from build123d import *

# Parameters (mm, degrees)
F0_W     = 75
F0_H     = 250
F1_DEPTH = 4
F2_W     = 40
F2_H     = 40
F3_DEPTH = 500
F4_W     = 30
F4_H     = 32
F5_DEPTH = 499
F6_R     = 5
F7_R     = 3
F9_DEPTH = 4


with BuildPart() as f1:
    # F0 (on Top) → F1 (new body)
    with BuildSketch(Plane.XY):
        with Locations((37.5, 125)):
            Rectangle(F0_W, F0_H)
    extrude(amount=F1_DEPTH)

    # F2 (on face) → F3 (join)
    with BuildSketch(Plane.XY.offset(4)):
        with Locations((37.5, 187.5)):
            Rectangle(F2_W, F2_H)
    extrude(amount=F3_DEPTH)

    # F4 (on face) → F5 (cut)
    with BuildSketch(Plane.XY.offset(504)):
        with Locations((37.5, 187.5)):
            Rectangle(F4_W, F4_H)
    extrude(amount=-F5_DEPTH, mode=Mode.SUBTRACT)

    # F6
    f6_edges = [f1.edges().sort_by_distance(p)[0] for p in [
        (57.5, 167.5, 254),
        (57.5, 207.5, 254),
        (17.5, 207.5, 254),
        (17.5, 167.5, 254),
    ]]
    fillet(f6_edges, radius=F6_R)

    # F7
    f7_edges = [f1.edges().sort_by_distance(p)[0] for p in [
        (0, 250, 2),
        (0, 0, 2),
        (75, 0, 2),
        (75, 250, 2),
    ]]
    fillet(f7_edges, radius=F7_R)

    # F8 (on face) → F9 (join)
    with BuildSketch(Plane.YZ.offset(57.5)):
        Polygon((172.5, 369.087671), (14.281406, 4), (44.281406, 4), (202.5, 369.087671), align=None)
    extrude(amount=F9_DEPTH)


solid = f1.part
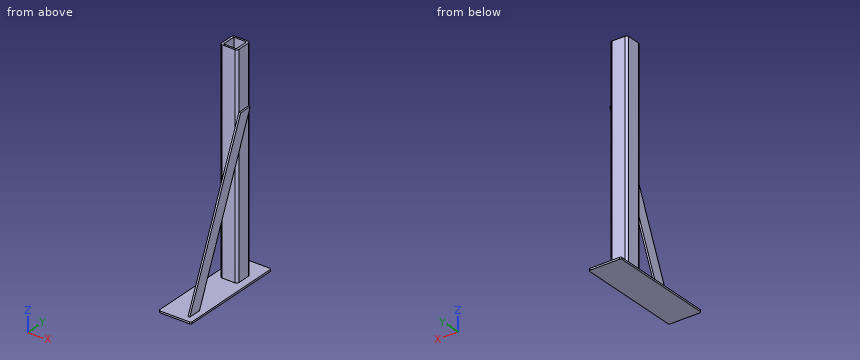
Could you check a few things on this model? Use its own coordinates, in mm. Round coordinates to 2 decimals unless told otherwise and drop trailing zeros. Loops run counter-clockwise (first coordinate to the right, second up) from the corner with the lowest first, then second, coordinate; pieces in that order, holes last. Notation, with made-up numbers: (22, 74) -> (65, 74) arc R31 ccw to (65, 110) -> close; hole circle Ø7 at (33, -31). An arc over 180 degrees is marked (long way). Use CSV: the item, a comma, the result in double quotes.
(1) If I drill on probe 1 along Y at (x, z) = (34, 323.5); probe 2 along Z at (x, y) = (51.5, 152.5); probe 3 along X at (y, z) = (58, 85), over which ranges is the centre line in solid material (lowest first)? Write a range as [from, to].
Return value:
probe 1,"y = [167.5, 171.5], [203.5, 207.5]"
probe 2,"z = [0, 4]"
probe 3,"x = [57.5, 61.5]"
(2) Suppose I cut it at C-C on y = 67. Write out the boundary of the cut face in (x, z), plus the area to 3 significant figures.
Return value:
outline,"(0, 0) -> (75, 0) -> (75, 4) -> (0, 4) -> close; (57.5, 56.42) -> (61.5, 56.42) -> (61.5, 125.65) -> (57.5, 125.65) -> close"
area,"577 mm²"
(3) Suppose I cut it at A-A on z = 54. Write out the boundary of the cut face in (x, y), plus the area to 3 significant figures.
Return value:
outline,"(17.5, 172.5) arc R5 ccw to (22.5, 167.5) -> (52.5, 167.5) arc R5 ccw to (57.5, 172.5) -> (57.5, 202.5) arc R5 ccw to (52.5, 207.5) -> (22.5, 207.5) arc R5 ccw to (17.5, 202.5) -> close; (57.5, 35.95) -> (61.5, 35.95) -> (61.5, 65.95) -> (57.5, 65.95) -> close; hole (22.5, 171.5) -> (52.5, 171.5) -> (52.5, 203.5) -> (22.5, 203.5) -> close"
area,"739 mm²"
(4) Suppose I cut it at B-B on x = 41. Write out the boundary of the cut face in (y, z), plus the area to 3 significant figures.
Return value:
outline,"(0, 0) -> (250, 0) -> (250, 4) -> (207.5, 4) -> (207.5, 504) -> (203.5, 504) -> (203.5, 5) -> (171.5, 5) -> (171.5, 504) -> (167.5, 504) -> (167.5, 4) -> (0, 4) -> close"
area,"5,030 mm²"
(5) Suppose I cut it at D-D on z = 472. Write out the boundary of the cut face in (x, y), plus the area to 3 significant figures.
Return value:
outline,"(17.5, 172.5) arc R5 ccw to (22.5, 167.5) -> (52.5, 167.5) arc R5 ccw to (57.5, 172.5) -> (57.5, 202.5) arc R5 ccw to (52.5, 207.5) -> (22.5, 207.5) arc R5 ccw to (17.5, 202.5) -> close; hole (22.5, 171.5) -> (52.5, 171.5) -> (52.5, 203.5) -> (22.5, 203.5) -> close"
area,"619 mm²"
(6) Will these pins go through, and if not, where does the flat tip stop? pin 1 Ø3 at (x, y) = (64.5, 185.5) entering from -Z; pin 2 Ø15 at (x, z) = (44.5, 353.5) entering from +Y; pin 3 Ø15 at (y, z) = (187.5, 151.5) entering from -X; pin 4 Ø5 at (y, z) = (208, 239.5) entering from -X.
Return value:
pin 1,"stops at z = 0"
pin 2,"stops at y = 207.5"
pin 3,"stops at x = 17.5"
pin 4,"stops at x = 18.5"
